from build123d import *

# Parameters (mm, degrees)
F1_DEPTH = 12.7
F2_SIZE2 = 12.69999
F2_SIZE  = 12.69999
F6_R     = 5.08


# Not quite as in the source:
# - a fillet or chamfer is up to 0.001 mm smaller than in the source, because OpenCascade refuses the exact size


with BuildPart() as f1:
    # F0 (on Top) → F1 (new body)
    with BuildSketch(Plane.XY):
        Polygon((-31.75, 13.1512806053), (-31.75, -13.1512806053), (-13.1512806053, -31.75), (13.1512806053, -31.75), (31.75, -13.1512806053), (31.75, 13.1512806053), (13.1512806053, 31.75), (-13.1512806053, 31.75), align=None)
    extrude(amount=F1_DEPTH)

    # F2 (size 12.7 and 12.7 in the source; OpenCascade refuses exactly that, so slightly less here)
    f2_edges = [f1.edges().sort_by_distance(p)[0] for p in [
        (-22.45064, 22.45064, 12.7),
        (-31.75, 0, 12.7),
        (-22.45064, -22.45064, 12.7),
        (0, -31.75, 12.7),
        (22.45064, -22.45064, 12.7),
        (31.75, 0, 12.7),
        (22.45064, 22.45064, 12.7),
        (0, 31.75, 12.7),
    ]]
    chamfer(f2_edges, length=F2_SIZE, length2=F2_SIZE2)

    # F1_face (on face) → F5 section 0
    with BuildSketch(Plane(origin=(0, 0, 0), x_dir=(1, 0, 0), z_dir=(0, 0, -1)), mode=Mode.PRIVATE) as f5_s0:
        Polygon((-31.75, -13.1512806053), (-13.1512806053, -31.75), (13.1512806053, -31.75), (31.75, -13.1512806053), (31.75, 13.1512806053), (13.1512806053, 31.75), (-13.1512806053, 31.75), (-31.75, 13.1512806053), align=None)
    loft([f5_s0.sketch, Vertex(0, 0, -50.8)])

    # F6
    f6_edges = [f1.edges().sort_by_distance(p)[0] for p in [
        (-13.470391, 13.470391, 12.7),
        (0, 19.05001, 12.7),
        (-19.05001, 0, 12.7),
        (13.470391, 13.470391, 12.7),
        (-13.470391, -13.470391, 12.7),
        (19.05001, 0, 12.7),
        (0, -19.05001, 12.7),
        (13.470391, -13.470391, 12.7),
        (-22.45064, 22.45064, 1e-05),
        (0, 31.75, 1e-05),
        (-31.75, 0, 0),
        (22.45064, 22.45064, 0),
        (-22.45064, -22.45064, 0),
        (31.75, 0, 0),
        (0, -31.75, 0),
        (22.45064, -22.45064, 0),
    ]]
    fillet(f6_edges, radius=F6_R)


solid = f1.part
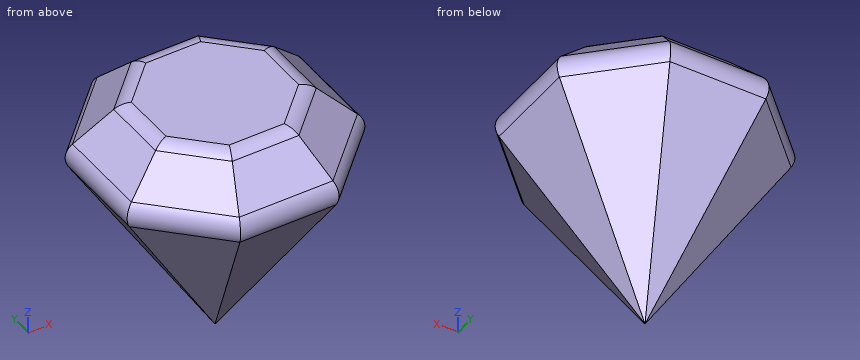
The listing builds one solid part. Answer for the finished solid, in the listing's coordinates (mm). Round coordinates to 2 decimals unless told otherwise and drop trailing zeros. Order: outer loops, then holes, each group sorted by start corner. A loop starts at its lowest first (then second) coordinate and runs counter-clockwise, first axis right, second up. Notation, with made-up numbers: M -26.75,-35.5 L 21.25,-35.5 A24 cw 21.25,-15.5 Z; hole C 53,-14 d1. An arc over 180 degrees is marked long. Answer in a Markdown table with one row per item. Add a question column.
1) The part is cut by section B-B on z = -9. Determine the outline of the cut face in (x, y) (3 decimals).
2) The part is cut by section C-C on y = 5.5. Determine the outline of the cut face in (x, z), plus the area to 3 significant figures.
3) Flat-ended cylindrical pins translate along their axes: pin 1 Ø4 at (x, y) = (0.5, -24) entering from -Z; pin 2 Ø12 at (x, z) = (23, -23.5) entering from +Y; pin 3 Ø12 at (x, z) = (22, -20) entering from -Y. Find the tip coordinate at first contact, or state that the pin passes through.
4) The part is cut by section D-D on z = -27. Determine the outline of the cut face in (x, y) (3 decimals).
5) The part is cut by section A-A on x = 5. Determine the outline of the cut face in (y, z), plus the area to 3 significant figures.
6) Consider line 1 along X through (y, z) = (19.5, -5); line 2 along X through (y, z) = (4.5, -29) (3 decimals); line 3 along Z through (x, y) = (8.5, -7.5). Determine where each line is inside the solid, lowest interval first. Write a range as from..to.
Findings below:
| question | item | result |
|---|---|---|
| 1 | outline | M -26.125,-10.821 L -10.821,-26.125 L 10.821,-26.125 L 26.125,-10.821 L 26.125,10.821 L 10.821,26.125 L -10.821,26.125 L -26.125,10.821 Z |
| 2 | outline | M -29.61,-3.43 L -13.28,-29.55 L -2.28,-42 L 2.28,-42 L 13.28,-29.55 L 29.61,-3.43 A5.08 ccw 28.89,2.86 L 20.54,11.21 A5.08 ccw 16.95,12.7 L -16.95,12.7 A5.08 ccw -20.54,11.21 L -28.89,2.86 A5.08 ccw Z |
| 2 | area | 2,160 mm² |
| 3 | pin 1 | stops at z = -15.6 |
| 3 | pin 2 | stops at y = 9.14 |
| 3 | pin 3 | stops at y = -13.23 |
| 4 | outline | M -14.875,-6.161 L -6.161,-14.875 L 6.161,-14.875 L 14.875,-6.161 L 14.875,6.161 L 6.161,14.875 L -6.161,14.875 L -14.875,6.161 Z |
| 5 | outline | M -29.61,-3.43 L -12.07,-31.49 L -2.07,-42.8 L 2.07,-42.8 L 12.07,-31.49 L 29.61,-3.43 A5.08 ccw 28.89,2.86 L 20.54,11.21 A5.08 ccw 16.95,12.7 L -16.95,12.7 A5.08 ccw -20.54,11.21 L -28.89,2.86 A5.08 ccw Z |
| 5 | area | 2,180 mm² |
| 6 | line 1 | x = -20.98..20.98 |
| 6 | line 2 | x = -13.625..13.625 |
| 6 | line 3 | z = -32.7..12.7 |
